CAD build for the part. Positions are in the model's coordinates, mm. A direction names the side the tool comes from. Give positions to 0.01 mm unless a question says otherwise; leave off trailing zeros. Write each loop counter-clockwise with the first axis right and the second up, starting at its lowest first coordinate (ties: lowest second). Pieces come first, ordered by that corner, then holes. Notation, with made-up numbers: (10.25, 8) -> (66.25, 8) arc R24 ccw to (66.25, 25) -> close; hole circle Ø4 at (45.25, -26.5). An arc over 180 degrees is marked (long way). Answer as a JSON object with one key per item and string values.
```python
from build123d import *

# Parameters (mm, degrees)
SKETCH002_R       = 3.35
SKETCH002_R_2     = 2.1
PAD002_DEPTH      = 10
SKETCH003_R       = 3.25
POCKET_DEPTH      = 15.001
POCKET_DEPTH_BACK = 15.001
SKETCH004_W       = 11
SKETCH004_H       = 11
POCKET001_DEPTH   = 7.5


with BuildPart() as part:
    # Sketch002 → Pad002 (new body)
    with BuildSketch(Plane.XY):
        with BuildLine():
            ThreePointArc((15, 0), (0, 15), (-15, 0))
            Line((-15, 0), (-15, -25))
            Line((-15, -25), (15, -25))
            Line((15, -25), (15, 0))
        make_face()
        Circle(SKETCH002_R, mode=Mode.SUBTRACT)
        with Locations((-6.914797, 6.914797)):
            Circle(SKETCH002_R_2, mode=Mode.SUBTRACT)
        with Locations((6.914797, 6.914797)):
            Circle(SKETCH002_R_2, mode=Mode.SUBTRACT)
        with Locations((6.914797, -6.914797)):
            Circle(SKETCH002_R_2, mode=Mode.SUBTRACT)
        with Locations((-6.914797, -6.914797)):
            Circle(SKETCH002_R_2, mode=Mode.SUBTRACT)
    extrude(amount=PAD002_DEPTH)

    # Sketch003 → Pocket (cut, two sides)
    with BuildSketch(Plane.YZ) as pocket_sk:
        with Locations((-20, 5)):
            Circle(SKETCH003_R)
        with BuildLine():
            ThreePointArc((-20, 10), (-25, 4.999992), (-19.999984, 0))
            Line((-26, 0), (-19.999984, 0))
            Line((-26, 10), (-26, 0))
            Line((-20, 10), (-26, 10))
        make_face()
    extrude(amount=-POCKET_DEPTH, mode=Mode.SUBTRACT)
    extrude(pocket_sk.sketch, amount=POCKET_DEPTH_BACK, mode=Mode.SUBTRACT)

    # Sketch004 → Pocket001 (cut, symmetric)
    with BuildSketch(Plane.YZ):
        with Locations((-19.5, 5.5)):
            Rectangle(SKETCH004_W, SKETCH004_H)
    extrude(amount=POCKET001_DEPTH, both=True, mode=Mode.SUBTRACT)


solid = part.part
```
1) Pin check, flat tips, straight feed: pin 1 (3 mm diameter, centred on y = 3, z = 5, fed in from -X); pin 2 (3 mm diameter, centred on x = 1.5, z = 5.5, fed in from -Y); pin 3 (1 mm diameter, centred on x = 2, z = 5.5, fed in from +Y). Stop position of each tip, or through.
Model answer:
{"pin 1": "stops at x = -14.92", "pin 2": "stops at y = -14", "pin 3": "stops at y = 14.92"}
2) Mould opens along Y. For faces 3 (the cylindrical face through (0, 15, 5)), 4 (the cylindrical face through (-11, -25, 5)), 5 (the cylindrical face through (-11.198, -23.247, 5.143)) say: released by +Y, released by -Y, zero draft, split by the parting line, or undercut.
Model answer:
{"face 3": "released by +Y", "face 4": "released by -Y", "face 5": "undercut"}
3) Slice it at B-B (z = 5). List the corners of the cut face in (x, y), then the cut area to 3 significant figures.
Model answer:
{"outline": "(-15, -25) -> (-7.5, -25) -> (-7.5, -23.25) -> (-15, -23.25) -> close; (-15, -16.75) -> (-7.5, -16.75) -> (-7.5, -14) -> (7.5, -14) -> (7.5, -16.75) -> (15, -16.75) -> (15, 0) arc R15 ccw to (-15, 0) -> close; (7.5, -25) -> (15, -25) -> (15, -23.25) -> (7.5, -23.25) -> close; hole circle Ø4.2 at (-6.91, -6.91); hole circle Ø4.2 at (-6.91, 6.91); hole circle Ø6.7 at (0, 0); hole circle Ø4.2 at (6.91, -6.91); hole circle Ø4.2 at (6.91, 6.91)", "area": "750 mm2"}
4) Slice it at A-A (x = -8.25). List the corners of the cut face in (y, z).
Model answer:
{"outline": "(-20, 0) -> (-8.54, 0) -> (-8.54, 10) -> (-20, 10) arc R5 ccw to start; (-5.29, 0) -> (5.29, 0) -> (5.29, 10) -> (-5.29, 10) -> close; (8.54, 0) -> (12.53, 0) -> (12.53, 10) -> (8.54, 10) -> close; hole circle Ø6.5 at (-20, 5)"}
5) Slice it at D-D (x = 0). List the corners of the cut face in (y, z), then the cut area to 3 significant figures.
Model answer:
{"outline": "(-14, 0) -> (-3.35, 0) -> (-3.35, 10) -> (-14, 10) -> close; (3.35, 0) -> (15, 0) -> (15, 10) -> (3.35, 10) -> close", "area": "223 mm2"}
6) 3-axis set-ups, long thin cutter, end or side, ignore diameter. For faces 1 (the flat face through (0, -14, 5)), 2 (the flat face through (3, -2, 0)): which of +Z, -Z, +X, -X, +Y, -Y reach the whole face in a straight line?
Model answer:
{"face 1": "+Z, -Z, -Y", "face 2": "-Z, +X, -X, +Y, -Y"}
7) Wall check: probe 1 along Y at (x, z) = (0, 4.5); probe 2 along X at (y, z) = (-5, 1.25); probe 3 along Y at (x, z) = (5.25, 5.5). Give the ranges that are in metal, low to high.
Model answer:
{"probe 1": "y = -14 to -3.35, 3.35 to 15", "probe 2": "x = -15 to -7.78, -6.05 to 6.05, 7.78 to 15", "probe 3": "y = -14 to -8.19, -5.63 to 5.63, 8.19 to 14.05"}
8) Slice it at C-C (y = 5.5). List the corners of the cut face in (x, z).
Model answer:
{"outline": "(-13.96, 0) -> (-8.47, 0) -> (-8.47, 10) -> (-13.96, 10) -> close; (-5.36, 0) -> (5.36, 0) -> (5.36, 10) -> (-5.36, 10) -> close; (8.47, 0) -> (13.96, 0) -> (13.96, 10) -> (8.47, 10) -> close"}
